For this review, take the finished solid that the model builds, in its own axes (mm). A direction names the side the tool comes from. Coordinates: 2 decimals unless noted, no trailing zeros. Loops run counter-clockwise (first coordinate to the right, second up) from the corner with the lowest first, then second, coordinate; pieces in that order, holes last. Notation, with made-up numbers: M 28,-32.5 L 73,-32.5 A15 cw 73,-9.5 Z; hole C 83.25,76.5 d5. An arc over 180 degrees is marked long. Answer as a JSON object with one key per item and string values. Group by question number.
Item 1: Add section C-C (y = -3). State the section outline as (x, z) points.
Item 2: Add section A-A (x = 0). State the section outline as (y, z) points (3 decimals), then the cut area to 3 significant figures.
Item 3: Mouldability with a two-part tool opening along X and no side actions: class faces 3 (the face through (-15.12, 4.7, 11.59)), 4 (the face through (-5, 0, -5)), 5 (the face through (1.17, -13.19, 4.83)) as +X half, -X half, draft (parallel to the pull), parting line (faces both ways), or undercut.
Item 4: Add section B-B (z = 0). State the section outline as (x, y) points (3 decimals), then the cut area to 3 significant figures.
Item 5: Wall thickness on L1, parallel to Z at x = 0, y = -10; L2, parallel to Y at x = 0, z = 4 (3 decimals); L3, parallel to Y at x = -16.5, z = -8 (3 decimals): over which ranges is each line inside the solid? List them lowest first. Write a range as from..to.
Item 6: Insertion check: pin 1 (1 mm diameter, centred on x = 0.5, z = 7.5, fed in from -Y); pin 2 (8 mm diameter, centred on y = 6.5, z = 15, fed in from +X); pin 3 (4 mm diameter, centred on y = -4.5, z = 0.5, fed in from +X). Each pin has a flat end and moves straight along its axis. Give the tip position at first contact, or say it passes through.
Item 7: Tool access review of faces 1 (the face through (0, 9.525, 0)), 2 (the face through (-1.38, -9.39, -6.2)): name each direction out of +Z, -Z, +X, -X, +Y, -Y from which nothing blocks a thin tool from reaching the whole face with its end or side.
Item 8: Add section D-D (y = 4.5). State the section outline as (x, z) points.
from build123d import *

# Parameters (mm, degrees)
SKETCH1_R           = 19.05
BOSS_EXTRUDE1_DEPTH = 9.525
SKETCH2_R           = 6.35
SKETCH2_R_2         = 3.5
BOSS_EXTRUDE2_DEPTH = 19.05
CUT_EXTRUDE1_REACH  = 27.4
SKETCH3_R           = 1.27


with BuildPart() as part:
    # Sketch1 → Boss-Extrude1 (new body)
    with BuildSketch(Plane(origin=(0, 0, 0), x_dir=(1, 0, 0), z_dir=(0, 1, 0))):
        Circle(SKETCH1_R)
    extrude(amount=BOSS_EXTRUDE1_DEPTH)

    # Sketch2 → Boss-Extrude2 (add)
    with BuildSketch(Plane.XZ):
        Circle(SKETCH2_R)
        Circle(SKETCH2_R_2, mode=Mode.SUBTRACT)
    extrude(amount=BOSS_EXTRUDE2_DEPTH)

    # Sketch3 → Cut-Extrude1 (cut, up to next)
    with BuildSketch(Plane.XY.offset(6.35), mode=Mode.PRIVATE) as cut_extrude1_sk1:
        with Locations((0, -12.7)):
            Circle(SKETCH3_R)
    cut_extrude1_tool1 = extrude(cut_extrude1_sk1.sketch, amount=-CUT_EXTRUDE1_REACH, mode=Mode.PRIVATE) & part.part
    add(cut_extrude1_tool1.solids().sort_by_distance((0, -12.7, 6.35))[0], mode=Mode.SUBTRACT)


solid = part.part
From the geometry:
{
 "1": {"outline": "C 0,0 d12.7; hole C 0,0 d7"},
 "2": {"outline": "M -19.05,-6.35 L 0,-6.35 L 0,-19.05 L 9.525,-19.05 L 9.525,19.05 L 0,19.05 L 0,6.35 L -11.43,6.35 L -11.43,3.5 L 0,3.5 L 0,-3.5 L -19.05,-3.5 Z; M -19.05,3.5 L -13.97,3.5 L -13.97,6.35 L -19.05,6.35 Z", "area": "464 mm²"},
 "3": {"face 3": "parting line", "face 4": "draft", "face 5": "undercut"},
 "4": {"outline": "M -19.05,0 L -6.35,0 L -6.35,-19.05 L -3.5,-19.05 L -3.5,0 L 3.5,0 L 3.5,-19.05 L 6.35,-19.05 L 6.35,0 L 19.05,0 L 19.05,9.525 L -19.05,9.525 Z", "area": "471 mm²"},
 "5": {"L1": "z = -6.35..-3.5, 3.5..6.35", "L2": "y = -19.05..-13.97, -11.43..9.525", "L3": "y = 0..9.525"},
 "6": {"pin 1": "stops at y = 0", "pin 2": "stops at x = 15.55", "pin 3": "stops at x = 6.35"},
 "7": {"face 1": "+Z, -Z, +X, -X, +Y", "face 2": "-Y"},
 "8": {"outline": "C 0,0 d38.1"}
}
